```python
from build123d import *

# Parameters (mm, degrees)
BASE_EXTRUDE_DEPTH = 3.175


with BuildPart() as part:
    # Sketch1 → Base-Extrude (new body)
    with BuildSketch(Plane.XY):
        with BuildLine():
            Line((-752.475, -70.85475791), (-701.6242, -339.127966514))
            ThreePointArc((-701.6242, -339.127966514), (0.43953811, -273.050025704), (702.4878, -339.292192091))
            Line((702.4878, -339.292192091), (752.475, -70.85475791))
            ThreePointArc((752.475, -70.85475791), (0, 0), (-752.475, -70.85475791))
        make_face()
        with BuildLine():
            Line((-501.033720833, -104.998443764), (-516.777000766, -156.384056801))
            add(Edge.make_bspline(
                [(-516.777000766, -156.384056801), (-543.069216838, -242.201094082), (-468.587308293, -233.583243234), (-394.105399749, -224.965392385), (-439.29934176, -147.419585798)],
                knots=[1.070267673, 1.070267673, 1.070267673, 3.141592654, 3.141592654, 5.212917634, 5.212917634, 5.212917634], degree=2, weights=[1, 0.50995617, 1, 0.50995617, 1]))
            Line((-439.29934176, -147.419585798), (-466.360616413, -100.986628705))
            ThreePointArc((-466.360616413, -100.986628705), (-485.00895367, -91.655109348), (-501.033720833, -104.998443764))
        make_face(mode=Mode.SUBTRACT)
    extrude(amount=-BASE_EXTRUDE_DEPTH)


solid = part.part
```
CAD build for the part. Positions are in the model's coordinates, mm. Coordinates: 2 decimals unless noted, no trailing zeros. Write each loop counter-clockwise with the first axis right and the second up, starting at its lowest first coordinate (ties: lowest second). Pieces come first, ordered by that corner, then holes. Notation, with made-up numbers: (30.5, -13) -> (86.5, -13) arc R9 ccw to (86.5, 2) -> close; hole circle Ø1 at (15.25, -27.75). An arc over 180 degrees is marked (long way). Use CSV: the item, a comma, the result in double quotes. Start each with the question number.
Item 1: Drop a flat-ended pin along its axis: P1, Ø1.5, axis at x = -230, z = -2.5, coming from the -Y side. Give the stop position or say it passes through.
Item 2: Two-plate mould, pull along X, no slides. Class faces 1 (the cylindrical face through (-9.45, -273.06, -1.57)), 2 (the cylindrical face through (10.597, -0.014, -1.565)), 3 (the flat face through (-11, -167, -3.175)), 4 (the flat face through (-452.64, -124.53, -1.57)): +X half, -X half, draft (parallel to the pull), parting line (faces both ways), or undercut.
Item 3: Band-saw the part on B-B, the plane x = -294.5. Write the cut outline in (y, z) (3 decimals).
Item 4: Band-saw the part on A-A, the plane y = -308.5. Write the cut outline in (x, z) (3 decimals).
Item 5: Wall check: probe 1 along X at (y, z) = (-105.5, -2.3); probe 2 along X at (y, z) = (-185.5, -1.15); probe 3 along Y at (x, z) = (437.5, -1.7). Give the ranges that are in metal, low to high.
Response values:
1,P1,"stops at y = -280.14"
2,face 1,"undercut"
2,face 2,"parting line"
2,face 3,"draft"
2,face 4,"undercut"
3,outline,"(-284.607, -3.175) -> (-10.772, -3.175) -> (-10.772, 0) -> (-284.607, 0) -> close"
4,outline,"(-707.43, -3.175) -> (-514.962, -3.175) -> (-514.962, 0) -> (-707.43, 0) -> close; (514.962, -3.175) -> (708.222, -3.175) -> (708.222, 0) -> (514.962, 0) -> close"
5,probe 1,"x = -745.91 to -501.19, -463.73 to 746.02"
5,probe 2,"x = -730.74 to -518.87, -430.49 to 731.13"
5,probe 3,"y = -298.6 to -23.81"
